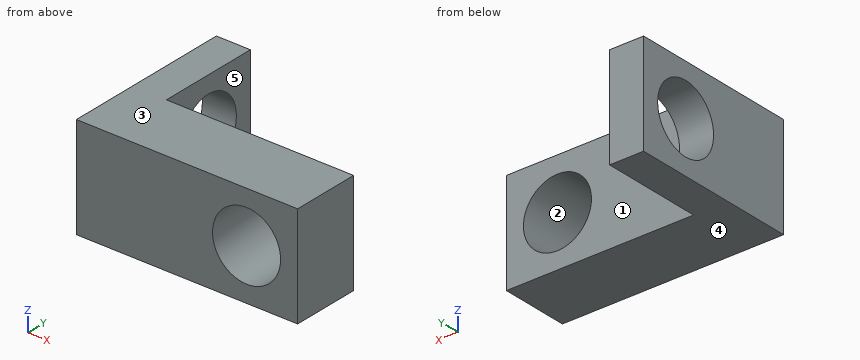
```python
from build123d import *

# Parameters (mm, degrees)
BOSS_EXTRUDE3_DEPTH = 30
SKETCH6_R           = 10
CUT_EXTRUDE2_DEPTH  = 30
SKETCH7_R           = 10
CUT_EXTRUDE3_DEPTH  = 30


with BuildPart() as part:
    # Sketch5 → Boss-Extrude3 (new body)
    with BuildSketch(Plane.XY):
        Polygon((0, 0), (0, 50), (10, 50), (10, 20), (65, 20), (65, 0), align=None)
    extrude(amount=-BOSS_EXTRUDE3_DEPTH)

    # Sketch6 → Cut-Extrude2 (cut)
    with BuildSketch(Plane(origin=(0, 20, 0), x_dir=(1, 0, 0), z_dir=(0, 1, 0))):
        with Locations(Location((50, 15, 0), (0, 0, 270))):
            Circle(SKETCH6_R)
    extrude(amount=-CUT_EXTRUDE2_DEPTH, mode=Mode.SUBTRACT)

    # Sketch7 → Cut-Extrude3 (cut)
    with BuildSketch(Plane(origin=(10, 0, 0), x_dir=(0, 0, -1), z_dir=(1, 0, 0))):
        with Locations(Location((15, 35, 0), (0, 0, 90))):
            Circle(SKETCH7_R)
    extrude(amount=-CUT_EXTRUDE3_DEPTH, mode=Mode.SUBTRACT)


solid = part.part
```
Check sheet for the modelled part. Datum: model origin and axes. Units: mm. Face numbers are marked on the shaded views. A direction names the side the tool comes from. Give positions to 0.01 mm unless a question says otherwise; leave off trailing zeros. Order: outer loops, then holes, each group sorted by start corner. A loop starts at its lowest first (then second) coordinate and runs counter-clockwise, first axis right, second up. Notation, with made-up numbers: (56.25, 51) -> (94.25, 51) arc R18 ccw to (94.25, 77) -> close; hole circle Ø5 at (11.5, 16). An arc over 180 degrees is marked (long way). Use CSV: the item, a comma, the result in double quotes. Start each with the question number.
1) Sectioned sample at B-B, the plane y = 35. Record the boundary of the cut face in (x, z), plus the area to 3 significant figures.
2) Mould release check, pull along Z, two halves, no side actions. Record for the marked faces 1, 2 and 3: released by +Z, released by -Z, zero draft, split by the parting line, or undercut.
3) Go/stop test with a flat-tipped pin: P1, Ø6, axis at x = 30, z = -25, coming from the +Y side. Record where the tip stops, or that it passes through.
4) Sectioned sample at A-A, the plane z = -15. Record the boundary of the cut face in (x, y), plus the area to 3 significant figures.
5) Sectioned sample at D-D, the plane z = -26. Record the boundary of the cut face in (x, y), plus the area to 3 significant figures.
6) Sectioned sample at C-C, the plane x = 50. Record the boundary of the cut face in (y, z).
7) Material ranges on line 1 (Z direction, x = 4.25, y = 35); line 2 (X direction, y = 5, z = -15); line 3 (Y direction, x = 11.5, z = -19), recorded low to high. Write a range as from..to.
8) Set-up check for the marked faces 4 and 5: record each of +Z, -Z, +X, -X, +Y, -Y from which the full face is reachable in a straight line by a thin tool's end or side.
Recorded:
1,outline,"(0, -30) -> (10, -30) -> (10, -25) -> (0, -25) -> close; (0, -5) -> (10, -5) -> (10, 0) -> (0, 0) -> close"
1,area,"100 mm2"
2,face 1,"zero draft"
2,face 2,"undercut"
2,face 3,"released by +Z"
3,P1,"y = 20"
4,outline,"(0, 0) -> (40, 0) -> (40, 20) -> (10, 20) -> (10, 25) -> (0, 25) -> close; (0, 45) -> (10, 45) -> (10, 50) -> (0, 50) -> close; (60, 0) -> (65, 0) -> (65, 20) -> (60, 20) -> close"
4,area,"1,000 mm2"
5,outline,"(0, 0) -> (65, 0) -> (65, 20) -> (10, 20) -> (10, 50) -> (0, 50) -> close"
5,area,"1,600 mm2"
6,outline,"(0, -30) -> (20, -30) -> (20, -25) -> (0, -25) -> close; (0, -5) -> (20, -5) -> (20, 0) -> (0, 0) -> close"
7,line 1,"-30..-25, -5..0"
7,line 2,"0..40, 60..65"
7,line 3,"0..20"
8,face 4,"-Z, +X, -X, +Y, -Y"
8,face 5,"+Z, -Z, +X, +Y"
